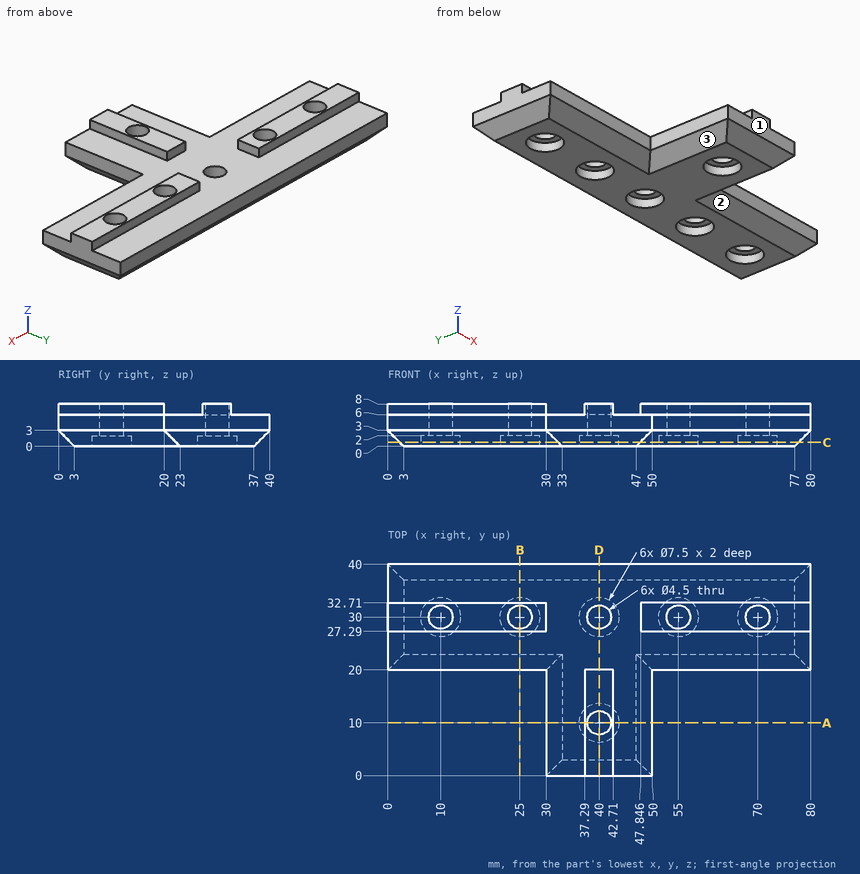
Answer from the drawing. Dimensions are ordinates in mm from the lowest x, y and z of the part. A direction names the side the tool comes from. Coordinates: 2 decimals unless noted, no trailing zeros. Loops run counter-clockwise (first coordinate to the right, second up) from the corner with the lowest first, then second, coordinate; pieces in that order, holes last. Notation, with made-up numbers: (79.5, 51) -> (133.5, 51) arc R26 cw to (133.5, 80) -> close; hole circle Ø9 at (79, 84). An arc over 180 degrees is marked (long way). Answer in a Markdown table with one row per item.
Item 1: Each of these flat-tipped pins is pushed along its axis until it touches: P1, Ø2.5, axis at x = 55, y = 30, coming from the +Z side; P2, Ø1, axis at x = 22, z = 7.5, coming from the +Y side; P3, Ø4, axis at x = 41, y = 28.5, coming from the -Z side; P4, Ø2.5, axis at x = 67, z = 5, coming from the -Y side. Where does it stop, or does it pass through?
Returned:
| item | result |
|---|---|
| P1 | passes through |
| P2 | stops at y = 32.71 |
| P3 | stops at z = 0 |
| P4 | stops at y = 20 |
Item 2: Straight lines are drawn through the part: line 1 along X through (y, z) = (30, 4.75); line 2 along Y through (x, z) = (40, 3.7); line 3 along X through (y, z) = (10, 5.25). For each, find the intervals that lie inside material, in ascending order. Write a range as [from, to].
Returned:
| item | result |
|---|---|
| line 1 | x = [0, 7.75], [12.25, 22.75], [27.25, 37.75], [42.25, 52.75], [57.25, 67.75], [72.25, 80] |
| line 2 | y = [0, 7.75], [12.25, 27.75], [32.25, 40] |
| line 3 | x = [30, 37.75], [42.25, 50] |
Item 3: A cutting plane is placed at C-C on z = 0.75. Determine the outline of the cut face in (x, y).
Returned:
| item | result |
|---|---|
| outline | (2.25, 22.25) -> (32.25, 22.25) -> (32.25, 2.25) -> (47.75, 2.25) -> (47.75, 22.25) -> (77.75, 22.25) -> (77.75, 37.75) -> (2.25, 37.75) -> close; hole circle Ø7.5 at (10, 30); hole circle Ø7.5 at (25, 30); hole circle Ø7.5 at (40, 10); hole circle Ø7.5 at (40, 30); hole circle Ø7.5 at (55, 30); hole circle Ø7.5 at (70, 30) |
Item 4: For the marked faces 1, 2 and 3, determine the directions among +Z, -Z, +X, -X, +Y, -Y from which every point of the face is accessible in a straight line to the end or side of a thin tool.
Returned:
| item | result |
|---|---|
| face 1 | +Z, -Z, +X, -X, -Y |
| face 2 | -Z, +X, -Y |
| face 3 | -Z, -X, -Y |
Item 5: A cutting plane is placed at B-B on x = 25. Determine the outline of the cut face in (y, z).
Returned:
| item | result |
|---|---|
| outline | (20, 3) -> (23, 0) -> (26.25, 0) -> (26.25, 2) -> (27.75, 2) -> (27.75, 8) -> (27.29, 8) -> (27.29, 6) -> (20, 6) -> close; (32.25, 2) -> (33.75, 2) -> (33.75, 0) -> (37, 0) -> (40, 3) -> (40, 6) -> (32.71, 6) -> (32.71, 8) -> (32.25, 8) -> close |
Item 6: A cutting plane is placed at D-D on x = 40. Determine the outline of the cut face in (y, z).
Returned:
| item | result |
|---|---|
| outline | (0, 3) -> (3, 0) -> (6.25, 0) -> (6.25, 2) -> (7.75, 2) -> (7.75, 8) -> (0, 8) -> close; (12.25, 2) -> (13.75, 2) -> (13.75, 0) -> (26.25, 0) -> (26.25, 2) -> (27.75, 2) -> (27.75, 6) -> (20, 6) -> (20, 8) -> (12.25, 8) -> close; (32.25, 2) -> (33.75, 2) -> (33.75, 0) -> (37, 0) -> (40, 3) -> (40, 6) -> (32.25, 6) -> close |
Item 7: A cutting plane is placed at A-A on y = 10. Determine the outline of the cut face in (x, z).
Returned:
| item | result |
|---|---|
| outline | (30, 3) -> (33, 0) -> (36.25, 0) -> (36.25, 2) -> (37.75, 2) -> (37.75, 8) -> (37.29, 8) -> (37.29, 6) -> (30, 6) -> close; (42.25, 2) -> (43.75, 2) -> (43.75, 0) -> (47, 0) -> (50, 3) -> (50, 6) -> (42.71, 6) -> (42.71, 8) -> (42.25, 8) -> close |
